```python
from build123d import *

# Parameters (mm, degrees)
ESQUISSE1_W                  = 140
ESQUISSE1_H                  = 35
BOSS_EXTRU_1_DEPTH           = 30
ESQUISSE2_W                  = 33
ESQUISSE2_H                  = 35
ENL_V_MAT_EXTRU_1_DEPTH      = 20
ESQUISSE3_W                  = 30
ESQUISSE3_H                  = 5
BOSS_EXTRU_2_DEPTH           = 30
ENL_V_MAT_EXTRU_2_DEPTH      = 149.660687473
ENL_V_MAT_EXTRU_2_DEPTH_BACK = 149.660687473
ESQUISSE4_R                  = 3
ENL_V_MAT_EXTRU_3_DEPTH      = 149.660687473
ENL_V_MAT_EXTRU_3_DEPTH_BACK = 149.660687473
ESQUISSE5_W                  = 65
ESQUISSE5_H                  = 2
ENL_V_MAT_EXTRU_4_DEPTH      = 149.660687473
ENL_V_MAT_EXTRU_4_DEPTH_BACK = 149.660687473
ESQUISSE6_W                  = 32
ESQUISSE6_H                  = 5
CONG_1_R                     = 3
ENL_V_MAT_EXTRU_6_DEPTH      = 15
ENL_V_MAT_EXTRU_5_DEPTH      = 149.660687473
ENL_V_MAT_EXTRU_5_DEPTH_BACK = 149.660687473
ESQUISSE7_R                  = 4
CONG_2_R                     = 3
CONG_3_R                     = 2
ENL_V_MAT_EXTRU_8_DEPTH      = 149.660687473
ENL_V_MAT_EXTRU_8_DEPTH_BACK = 149.660687473
ESQUISSE10_R                 = 3
ESQUISSE9_W                  = 140
ESQUISSE9_H                  = 40
ENL_V_MAT_EXTRU_7_DEPTH      = 20


with BuildPart() as part:
    # Esquisse1 → Boss.-Extru.1 (new body)
    with BuildSketch(Plane.XY):
        with Locations((70, 17.5)):
            Rectangle(ESQUISSE1_W, ESQUISSE1_H)
    extrude(amount=BOSS_EXTRU_1_DEPTH)

    # Esquisse2 → Enlèv. mat.-Extru.1 (cut)
    with BuildSketch(Plane.XY.offset(30)):
        with Locations((25, 17.5)):
            Rectangle(ESQUISSE2_W, ESQUISSE2_H)
    extrude(amount=-ENL_V_MAT_EXTRU_1_DEPTH, mode=Mode.SUBTRACT)

    # Esquisse3 → Boss.-Extru.2 (add)
    with BuildSketch(Plane.XY.offset(30)):
        with Locations((125, 37.5)):
            Rectangle(ESQUISSE3_W, ESQUISSE3_H)
    extrude(amount=-BOSS_EXTRU_2_DEPTH)

    # Esquisse4 → Enlèv. mat.-Extru.2 (cut, two sides: drawn at the far end of the back side and taken through both)
    with BuildSketch(Plane.XY.offset(30).offset(-ENL_V_MAT_EXTRU_2_DEPTH_BACK)):
        with Locations((75, 25)):
            Circle(ESQUISSE4_R)
    extrude(amount=ENL_V_MAT_EXTRU_2_DEPTH + ENL_V_MAT_EXTRU_2_DEPTH_BACK, mode=Mode.SUBTRACT)

    # Esquisse5 → Enlèv. mat.-Extru.3 (cut, two sides: drawn at the far end of the back side and taken through both)
    with BuildSketch(Plane.XY.offset(30).offset(-ENL_V_MAT_EXTRU_3_DEPTH_BACK)):
        with Locations((107.5, 25)):
            Rectangle(ESQUISSE5_W, ESQUISSE5_H)
    extrude(amount=ENL_V_MAT_EXTRU_3_DEPTH + ENL_V_MAT_EXTRU_3_DEPTH_BACK, mode=Mode.SUBTRACT)

    # Esquisse6 → Enlèv. mat.-Extru.4 (cut, two sides: drawn at the far end of the back side and taken through both)
    with BuildSketch(Plane.XY.offset(30).offset(-ENL_V_MAT_EXTRU_4_DEPTH_BACK)):
        with Locations((94, 32.5)):
            Rectangle(ESQUISSE6_W, ESQUISSE6_H)
    extrude(amount=ENL_V_MAT_EXTRU_4_DEPTH + ENL_V_MAT_EXTRU_4_DEPTH_BACK, mode=Mode.SUBTRACT)

    # Congé1
    cong_1_edges = [part.edges().sort_by_distance(p)[0] for p in [
        (78, 30, 15),
        (110, 30, 15),
    ]]
    fillet(cong_1_edges, radius=CONG_1_R)

    # Esquisse8 → Enlèv. mat.-Extru.6 (cut)
    with BuildSketch(Plane.XY.offset(30)):
        Polygon((72, 0), (140, 0), (140, 24), (106.275552162, 24), align=None)
    extrude(amount=-ENL_V_MAT_EXTRU_6_DEPTH, mode=Mode.SUBTRACT)

    # Esquisse7 → Enlèv. mat.-Extru.5 (cut, two sides: drawn at the far end of the back side and taken through both)
    with BuildSketch(Plane.XY.offset(30).offset(-ENL_V_MAT_EXTRU_5_DEPTH_BACK)):
        with Locations((125, 15)):
            Circle(ESQUISSE7_R)
    extrude(amount=ENL_V_MAT_EXTRU_5_DEPTH + ENL_V_MAT_EXTRU_5_DEPTH_BACK, mode=Mode.SUBTRACT)

    # Congé2
    cong_2_edges = [part.edges().sort_by_distance(p)[0] for p in [
        (140, 0, 7.5),
        (72, 0, 22.5),
        (0, 35, 15),
        (0, 0, 15),
    ]]
    fillet(cong_2_edges, radius=CONG_2_R)

    # Congé3
    cong_3_edges = [part.edges().sort_by_distance(p)[0] for p in [
        (106.275552162, 24, 22.5),
        (8.5, 0, 20),
        (8.5, 35, 20),
        (41.5, 35, 20),
        (41.5, 0, 20),
        (110, 40, 15),
        (140, 40, 15),
        (140, 26, 15),
        (140, 24, 7.5),
        (78, 35, 15),
    ]]
    fillet(cong_3_edges, radius=CONG_3_R - 0.0001)  # a hair under: the kernel refuses the full size

    # Esquisse10 → Enlèv. mat.-Extru.8 (cut, two sides: drawn at the far end of the back side and taken through both)
    with BuildSketch(Plane.XY.offset(30).offset(-ENL_V_MAT_EXTRU_8_DEPTH_BACK)):
        with Locations((56.5, 15)):
            Circle(ESQUISSE10_R)
        with Locations((125, 33)):
            Circle(ESQUISSE10_R)
    extrude(amount=ENL_V_MAT_EXTRU_8_DEPTH + ENL_V_MAT_EXTRU_8_DEPTH_BACK, mode=Mode.SUBTRACT)

    # Esquisse9 → Enlèv. mat.-Extru.7 (cut)
    with BuildSketch(Plane.XY.offset(30)):
        with Locations((70, 20)):
            Rectangle(ESQUISSE9_W, ESQUISSE9_H)
    extrude(amount=-ENL_V_MAT_EXTRU_7_DEPTH, mode=Mode.SUBTRACT)


solid = part.part
```
Input: part model. Units: mm. Frame: model coordinates. A direction names the side the tool comes from. Round coordinates to 2 decimals unless told otherwise and drop trailing zeros. Loops run counter-clockwise (first coordinate to the right, second up) from the corner with the lowest first, then second, coordinate; pieces in that order, holes last. Notation, with made-up numbers: M 7,40 L 29,40 A29 ccw 29,64 Z; hole C -13,-17.5 d7. An arc over 180 degrees is marked long. Answer in a Markdown table with one row per item. Add a question column.
1. Set-up query: faces 1 (the face through (39, 35, 5)), 2 (the face through (127.86, 33.9, 4.93)), 3 (the face through (140, 12, 5)), 4 (the face through (107, 26, 5)), 5 (the face through (110, 35, 5)). Return all of +Z, -Z, +X, -X, +Y, -Y with unobstructed straight access to the full face (end or side cutting, diameter ignored); none if empty.
2. Ray query, probe 1 along X at (y, z) = (15, 4); probe 2 along Y at (x, z) = (125, 3.5); probe 3 along Y at (x, z) = (56.5, 4.25). Return the intervals inside material, ascending.
3. Section D-D (x = 108.5). Output: boundary loops of the cut face in (y, z).
4. Section A-A (y = 15). Output: boundary loops of the cut face in (x, z).
5. Section C-C (x = 125). Output: boundary loops of the cut face in (y, z), and give its area (3 significant figures).
6. Mould query, pull axis X, two halves, no side actions, for faces 6 (the face through (69, 16, 10)), 7 (the face through (122.05, 17.7, 4.93)), 8 (the face through (72, 25, 5)), 9 (the face through (0.9, 0.86, 5.07)). Classes: released by +X, released by -X, zero draft, split by the parting line, or undercut.
7. Contact query for flat-ended pins moving along their axis: pin 1 (4 mm diameter, centred on y = 36.5, z = 3, fed in from -X); pin 2 (1 mm diameter, centred on x = 79, z = 2.5, fed in from +Y); pin 3 (5 mm diameter, centred on x = 48.5, z = 4.5, fed in from +Y). Output: stop coordinate, or through.
8. Section B-B (z = 6.25). Give the number of separate pieces and of enclosed holes in the cut face, and give its area (3 significant figures).
Values follow:
| question | item | result |
|---|---|---|
| 1 | face 1 | +Z, -Z, -X, +Y |
| 1 | face 2 | +Z, -Z |
| 1 | face 3 | +Z, -Z, +X, +Y, -Y |
| 1 | face 4 | +Z, -Z, +X |
| 1 | face 5 | +Z, -Z, +Y |
| 2 | probe 1 | 0 to 53.5, 59.5 to 121, 129 to 140 |
| 2 | probe 2 | 0 to 11, 19 to 24, 26 to 30, 36 to 40 |
| 2 | probe 3 | 0 to 12, 18 to 35 |
| 3 | outline | M 0,0 L 24,0 L 24,10 L 0,10 Z; M 26,0 L 30.4,0 L 30.4,10 L 26,10 Z |
| 4 | outline | M 0,0 L 53.5,0 L 53.5,10 L 0,10 Z; M 59.5,0 L 121,0 L 121,10 L 59.5,10 Z; M 129,0 L 140,0 L 140,10 L 129,10 Z |
| 5 | outline | M 0,0 L 11,0 L 11,10 L 0,10 Z; M 19,0 L 24,0 L 24,10 L 19,10 Z; M 26,0 L 30,0 L 30,10 L 26,10 Z; M 36,0 L 40,0 L 40,10 L 36,10 Z |
| 5 | area | 240 mm^2 |
| 6 | face 6 | zero draft |
| 6 | face 7 | undercut |
| 6 | face 8 | undercut |
| 6 | face 9 | released by -X |
| 7 | pin 1 | x = 1.34 |
| 7 | pin 2 | y = 31.34 |
| 7 | pin 3 | y = 35 |
| 8 | separate pieces | 1 |
| 8 | enclosed holes | 3 |
| 8 | area | 4,620 mm^2 |
